from build123d import *

# Parameters (mm, degrees)
SKETCH1_R           = 7.62
BOSS_EXTRUDE1_DEPTH = 660.4
SKETCH2_W           = 25.4
SKETCH2_H           = 38.1


with BuildPart() as part:
    # Sketch1 → Boss-Extrude1 (new body)
    with BuildSketch(Plane.XY):
        Circle(SKETCH1_R)
    extrude(amount=BOSS_EXTRUDE1_DEPTH)

    # Sketch2 → Revolve1 (revolve)
    with BuildSketch(Plane(origin=(0, 0, 0), x_dir=(1, 0, 0), z_dir=(0, 1, 0)), mode=Mode.PRIVATE) as revolve1_sk:
        with Locations((12.7, -127)):
            Rectangle(SKETCH2_W, SKETCH2_H)
        with Locations((12.7, -215.9)):
            Rectangle(SKETCH2_W, SKETCH2_H)
        with Locations((12.7, -432.054)):
            Rectangle(SKETCH2_W, SKETCH2_H)
        with Locations((12.7, -520.954)):
            Rectangle(SKETCH2_W, SKETCH2_H)
    revolve(revolve1_sk.sketch.rotate(Axis((0, 0, 0), (0, 0, 1)), 180), axis=Axis((0, 0, 0), (0, 0, 1)))


solid = part.part
Here's how the part is built. I have some questions about the finished solid (model axes, mm). A direction names the side the tool comes from. Round coordinates to 2 decimals unless told otherwise and drop trailing zeros. Loops run counter-clockwise (first coordinate to the right, second up) from the corner with the lowest first, then second, coordinate; pieces in that order, holes last. Notation, with made-up numbers: (69, 22.25) -> (109, 22.25) arc R29 cw to (109, 44.25) -> close; hole circle Ø3 at (-19, 80.5). An arc over 180 degrees is marked (long way). Write each question's results on one line, items separated by ' | '.
(1) If I drill on L1, parallel to Z at x = 7, y = -17.5; L2, parallel to Y at x = 0.5, z = 447.5; L3, parallel to X at y = 6.5, z = 118.5, over which ranges is the centre line in solid material (lowest first)?
Worked answers:
L1: 107.95 to 146.05, 196.85 to 234.95, 413 to 451.1, 501.9 to 540 | L2: -25.4 to 25.4 | L3: -24.55 to 24.55
(2) If we section it at A-A, the plane y = 19.5: List the corners of the cut face in (x, z) for me, then the cut area to 3 significant figures.
Worked answers:
outline: (-16.28, 107.95) -> (16.28, 107.95) -> (16.28, 146.05) -> (-16.28, 146.05) -> close; (-16.28, 196.85) -> (16.28, 196.85) -> (16.28, 234.95) -> (-16.28, 234.95) -> close; (-16.28, 413) -> (16.28, 413) -> (16.28, 451.1) -> (-16.28, 451.1) -> close; (-16.28, 501.9) -> (16.28, 501.9) -> (16.28, 540) -> (-16.28, 540) -> close | area: 4,960 mm2
(3) If we section it at B-B, the plane x = -17: List the corners of the cut face in (y, z) for me.
Worked answers:
outline: (-18.87, 107.95) -> (18.87, 107.95) -> (18.87, 146.05) -> (-18.87, 146.05) -> close; (-18.87, 196.85) -> (18.87, 196.85) -> (18.87, 234.95) -> (-18.87, 234.95) -> close; (-18.87, 413) -> (18.87, 413) -> (18.87, 451.1) -> (-18.87, 451.1) -> close; (-18.87, 501.9) -> (18.87, 501.9) -> (18.87, 540) -> (-18.87, 540) -> close
(4) We'd pull the mould along Z, two halves only. Please class faces 5 (the face through (5, -6, 107.95)), 6 (the face through (5, -6, 501.904)), 7 (the face through (0, 0, 660.4)): released by +Z, released by -Z, zero draft, split by the parting line, or undercut.
Worked answers:
face 5: released by -Z | face 6: undercut | face 7: released by +Z
(5) If we section it at C-C, the plane z = 570: List the corners of the cut face in (x, y) for me, then the cut area to 3 significant figures.
Worked answers:
outline: circle Ø15.24 at (0, 0) | area: 182 mm2
(6) For P1, Ø8, axis at x = 15, y = -10.5, coming from the -Z side; P2, Ø1.5, axis at y = -3.5, z = 363, coming from the +X side; P3, Ø6, axis at y = -5, z = 235, coming from the +X side, each with a flat end and sliding along its axis, tell me the tip position at first contact or that it passes through.
Worked answers:
P1: z = 107.95 | P2: x = 7.11 | P3: x = 25.32
(7) If we section it at D-D, the plane z = 217: List the corners of the cut face in (x, y) for me, then the cut area to 3 significant figures.
Worked answers:
outline: circle Ø50.8 at (0, 0) | area: 2,030 mm2
(8) For faces 1 (the face through (5, -6, 451.104)), 2 (the face through (5, -6, 540.004)), 3 (the face through (-11.721, 22.534, 215.633)), 4 (the face through (-1.65, -7.44, 53.22)), which set-ups out of +Z, -Z, +X, -X, +Y, -Y let a thin tool reach every point of the face, with its end or its side?
Worked answers:
face 1: none | face 2: +Z | face 3: +Z, -Z | face 4: -Z
